Part print with two shaded views. Sizes in mm from the minimum x, y, z corner. A direction names the side the tool comes from. Round coordinates to 2 decimals unless told otherwise and drop trailing zeros. Loops run counter-clockwise (first coordinate to the right, second up) from the corner with the lowest first, then second, coordinate; pieces in that order, holes last. Notation, with made-up numbers: (66, 88) - (124, 88) arc R34 ccw to (124, 121) - close; hole circle Ø10 at (79, -18). An arc over 180 degrees is marked (long way). One line per question, with ' | ' between items.
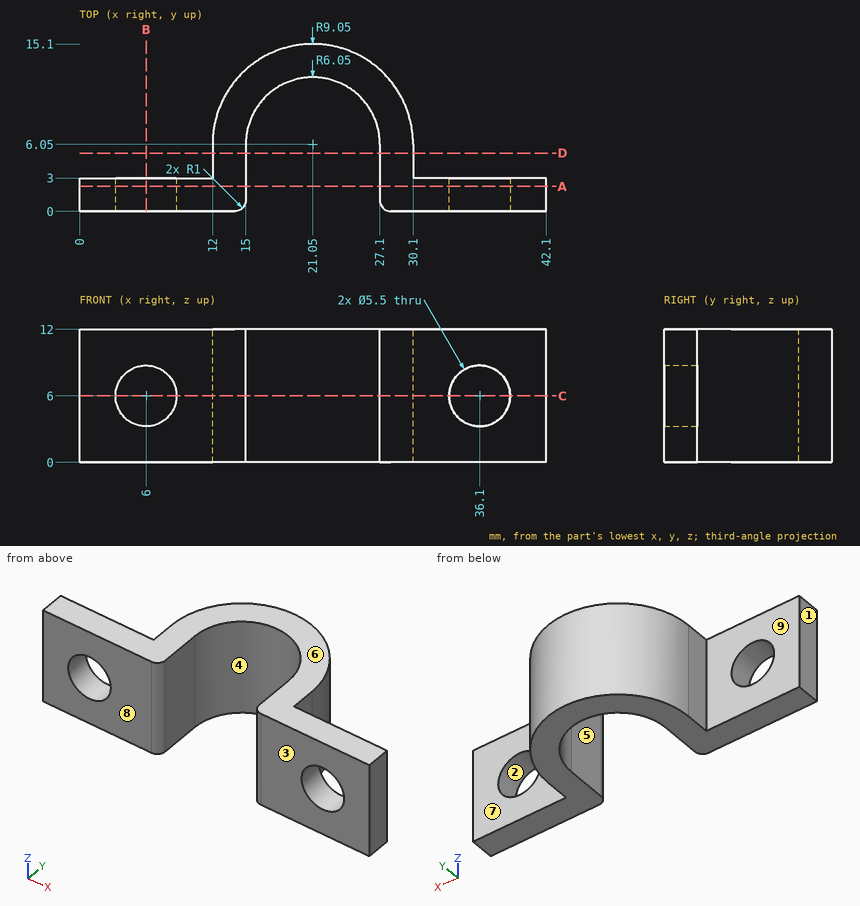
(1) Cut at B-B, the plane x = 6. Write the cut outline in (y, z).
Results found:
outline: (0, 0) - (3, 0) - (3, 3.25) - (0, 3.25) - close; (0, 8.75) - (3, 8.75) - (3, 12) - (0, 12) - close
(2) Probe L1, parallel to X at y = 1.45, z = 6; L2, parallel to Z at x = 36.1, y = 1; L3, parallel to X at y = 5, z = 2.75. List the from-to ranges inside material, lowest first.
Results found:
L1: x = 0 to 3.25, 8.75 to 15, 27.1 to 33.35, 38.85 to 42.1 | L2: z = 0 to 3.25, 8.75 to 12 | L3: x = 12 to 15, 27.1 to 30.1
(3) Cut at D-D, the plane y = 5.25. Write the cut outline in (x, z).
Results found:
outline: (12, 0) - (15, 0) - (15, 12) - (12, 12) - close; (27.1, 0) - (30.1, 0) - (30.1, 12) - (27.1, 12) - close
(4) Drop flat-ended pins along their axis: P1, Ø5, axis at y = 8.5, z = 3, coming from the -X side; P2, Ø6, axis at x = 5.5, z = 5, coming from the +Y side; P3, Ø1.5, axis at y = 4.5, z = 3, coming from the +X side. Give the stop position or say it passes through.
Results found:
P1: stops at x = 12 | P2: stops at y = 3 | P3: stops at x = 30.1
(5) Two-plate mould, pull along X, no slides. Class the marked faces 1, 2, 3 and 4: released by +X, released by -X, zero draft, split by the parting line, or undercut.
Results found:
face 1: released by -X | face 2: undercut | face 3: zero draft | face 4: undercut
(6) Cut at C-C, the plane z = 6. Write the cut outline in (x, y).
Results found:
outline: (0, 0) - (3.25, 0) - (3.25, 3) - (0, 3) - close; (8.75, 0) - (14, 0) arc R1 ccw to (15, 1) - (15, 6.05) arc R6.05 cw to (27.1, 6.05) - (27.1, 1) arc R1 ccw to (28.1, 0) - (33.35, 0) - (33.35, 3) - (30.1, 3) - (30.1, 6.05) arc R9.05 ccw to (12, 6.05) - (12, 3) - (8.75, 3) - close; (38.85, 0) - (42.1, 0) - (42.1, 3) - (38.85, 3) - close
(7) Cut at A-A, the plane y = 2.25. Write the cut outline in (x, z), then the cut area to 3 significant figures.
Results found:
outline: (0, 0) - (15, 0) - (15, 12) - (0, 12) - close; (27.1, 0) - (42.1, 0) - (42.1, 12) - (27.1, 12) - close; hole circle Ø5.5 at (6, 6); hole circle Ø5.5 at (36.1, 6) | area: 312 mm²
(8) Tool access for the marked faces 5, 6, 7, 8 and 9: list every direction of +Z, -Z, +X, -X, +Y, -Y with a clear straight run to the whole face (end or side of a thin tool).
Results found:
face 5: +Z, -Z, -Y | face 6: +Z, +X, -X, +Y, -Y | face 7: +Z, -Z, +X, +Y | face 8: +Z, -Z, +X, -X, -Y | face 9: +Z, -Z, -X, +Y
